```python
from build123d import *


with BuildPart() as part:
    # 草图1 → 旋转4 (revolve)
    with BuildSketch(Plane(origin=(0, 0, 0), x_dir=(0, 0, -1), z_dir=(1, 0, 0)), mode=Mode.PRIVATE) as revolve_4_sk:
        with BuildLine():
            Line((-7, 0), (0, 0))
            Line((0, 0), (0, 88))
            Line((0, 88), (-4.914147633, 88))
            ThreePointArc((-4.914147633, 88), (-6.328361195, 87.414213562), (-6.914147633, 86))
            Line((-6.914147633, 86), (-6.914147633, 82.933330123))
            Line((-6.914147633, 82.933330123), (-6.309364611, 82.933330123))
            Line((-6.309364611, 82.933330123), (-6.309364611, 80.780984357))
            Line((-6.309364611, 80.780984357), (-6.960648153, 80.780984357))
            Line((-6.960648153, 80.780984357), (-6.960648153, 77.82908336))
            Line((-6.960648153, 77.82908336), (-6.309364611, 77.82908336))
            Line((-6.309364611, 77.82908336), (-6.309364611, 75.328381362))
            Line((-6.309364611, 75.328381362), (-7.5, 75.328381362))
            Line((-7.5, 75.328381362), (-7.5, 46.447151695))
            Line((-7.5, 46.447151695), (-6.309364611, 46.447151695))
            Line((-6.309364611, 46.447151695), (-6.309364611, 43.835644878))
            Line((-6.309364611, 43.835644878), (-7, 43.835644878))
            Line((-7, 43.835644878), (-7, 0))
        make_face()
    revolve(revolve_4_sk.sketch.rotate(Axis((0, 0, 0), (0, 1, 0)), 180), axis=Axis((0, 0, 0), (0, 1, 0)))


solid = part.part
```
Geometry check sheet. Reference: the model listing, model coordinates, mm. A direction names the side the tool comes from. Round coordinates to 2 decimals unless told otherwise and drop trailing zeros. Loops run counter-clockwise (first coordinate to the right, second up) from the corner with the lowest first, then second, coordinate; pieces in that order, holes last. Notation, with made-up numbers: (36, 45.5) - (82, 45.5) arc R20 ccw to (82, 55.5) - close; hole circle Ø8 at (6.5, 83). An arc over 180 degrees is marked (long way). Write item = value, one per line. Start each with the question number.
1. Mould release check, pull along Y, two halves, no side actions. Record for faces 1 (the face through (-6.324, 60.686, -4.032)), 2 (the face through (-1.895, 76.561, -6.018)), 3 (the face through (0, 0, 0)): released by +Y, released by -Y, zero draft, split by the parting line, or undercut.
2. Section check C-C on y = 71. Enter the section's corners in (x, z), then the cut area to 3 significant figures.
3. Depth check by flat-ended pin: pin 1 (4 mm diameter, centred on x = 1, y = 21, fed in from -Z); pin 2 (5 mm diameter, centred on x = -5.5, y = 60.5, fed in from +Z); pin 3 (1.5 mm diameter, centred on y = 26.5, z = 2, fed in from +X); pin 4 (1.5 mm diameter, centred on x = 2.5, z = 4.5, fed in from -Y). Enter the tip coordinate at first touch or a pass-through.
4. Thickness scan on line 1 (Z direction, x = -3, y = 10); line 2 (X direction, y = 58, z = 0.5); line 3 (Z direction, x = -1, y = 25). Record the ranges inside material, lowest first.
5. Set-up check for faces 4 (the face through (0, 88, 0)), 5 (the face through (4.207, 84.445, 5.487)), 6 (the face through (6, 82.933, -3)), 7 (the face through (2.681, 21.611, -6.466)): record each of +Z, -Z, +X, -X, +Y, -Y from which the full face is reachable in a straight line by a thin tool's end or side.
6. Section check D-D on y = 32. Enter the section's corners in (x, z).
Working result:
q1.face_1 = zero draft
q1.face_2 = undercut
q1.face_3 = released by -Y
q2.outline = circle Ø15 at (0, 0)
q2.area = 177 mm^2
q3.pin_1 = -7
q3.pin_2 = 6.87
q3.pin_3 = 6.89
q3.pin_4 = 0
q4.line_1 = -6.32 to 6.32
q4.line_2 = -7.48 to 7.48
q4.line_3 = -6.93 to 6.93
q5.face_4 = +Z, -Z, +X, -X, +Y
q5.face_5 = +Y
q5.face_6 = none
q5.face_7 = -Y
q6.outline = circle Ø14 at (0, 0)
